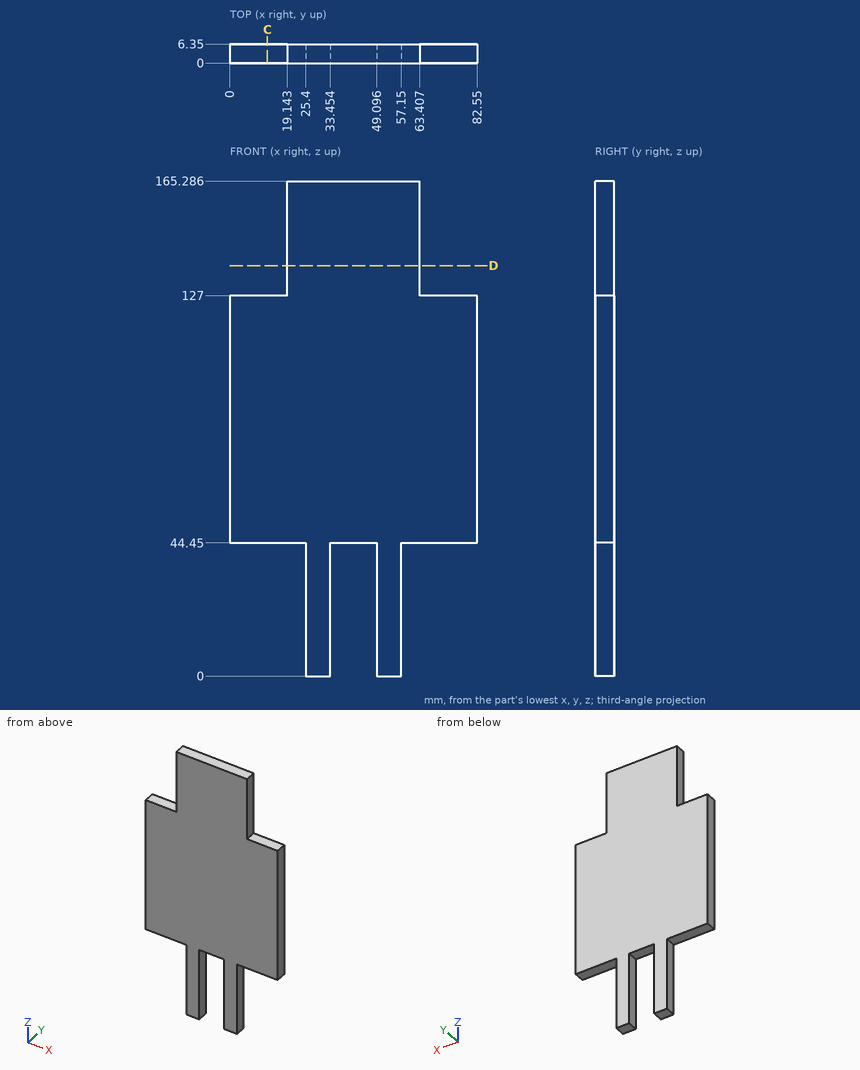
Could you check a few things on this drawing? It's one solid part, dimensions in mm from its lowest x, y, z. Coordinates: 2 decimals unless noted, no trailing zeros. Loops run counter-clockwise (first coordinate to the right, second up) from the corner with the lowest first, then second, coordinate; pieces in that order, holes last. Notation, with made-up numbers: (41.25, -21) - (90.25, -21) arc R15 cw to (90.25, -15) - close; hole circle Ø5 at (-5.5, 1). An arc over 180 degrees is marked (long way). Answer as a JSON object with one key per item and string values. Group by question number.
Item 1: If I drill on L1, parallel to Z at x = 46, y = 2.5; L2, parallel to X at y = 3, z = 147.5; L3, parallel to Z at x = 73.5, y = 5, over which ranges is the centre line in solid material (lowest first)? Write a range as from..to.
Item 2: For pin 1 (3 mm diameter, centred on x = 15.5, y = 3.5, fed in from -Z); pin 2 (1.9 mm diameter, centred on x = 68.5, y = 3, fed in from +Z); pin 3 (1.9 mm diameter, centred on y = 3, z = 19.5, fed in from +X), each with a flat end and sliding along its axis, tell me the tip position at first contact or that it passes through.
Item 3: If we section it at D-D (z = 137): List the corners of the cut face in (x, y) for me.
Item 4: If we section it at C-C (x = 12.5): List the corners of the cut face in (y, z) for me.
Returned:
{
 "1": {"L1": "z = 44.45..165.29", "L2": "x = 19.14..63.41", "L3": "z = 44.45..127"},
 "2": {"pin 1": "stops at z = 44.45", "pin 2": "stops at z = 127", "pin 3": "stops at x = 57.15"},
 "3": {"outline": "(19.14, 0) - (63.41, 0) - (63.41, 6.35) - (19.14, 6.35) - close"},
 "4": {"outline": "(0, 44.45) - (6.35, 44.45) - (6.35, 127) - (0, 127) - close"}
}
